Input: part model. Units: mm. Frame: model coordinates. A direction names the side the tool comes from. Coordinates: 2 decimals unless noted, no trailing zeros. Write each loop counter-clockwise with the first axis right and the second up, starting at its lowest first coordinate (ties: lowest second). Pieces come first, ordered by that corner, then holes. Notation, with made-up numbers: (-9.5, 11) -> (28.5, 11) arc R22 cw to (28.5, 34) -> close; hole circle Ø7 at (32.25, 29.5). An arc over 180 degrees is marked (long way). Use one line per item in the form item = value. Start each with the question number.
(1) Cut plane C-C on x = 5. Return the cut outline in (y, z) (3 decimals), plus the area to 3 significant figures.
(2) First-contact query: pin 1 (3 mm diameter, centred on x = 130, y = -77, fed in from +Z); pin 2 (9.5 mm diameter, centred on x = -242.5, z = 11, fed in from +Y); pin 3 (2 mm diameter, centred on x = 47.5, z = 30, fed in from -Y) (3 decimals); pin 4 (10 mm diameter, centred on x = 128, y = 30, fed in from -Z). Flat tips, straight axial feed; report the tip coordinate or a pass-through.
(3) Cut plane D-D on y = 0. Return the cut outline in (x, z).
(4) Cut plane B-B on x = 252. Return the cut outline in (y, z) (3 decimals), plus the area to 3 significant figures.
(5) Set-up query: faces 1 (the face through (-236, -92, 3.302)), 2 (the face through (-238.123, -85.516, 9.741)), 3 (the face through (177.8, 114, 28)). Return all of +Z, -Z, +X, -X, +Y, -Y with unobstructed straight access to the full face (end or side cutting, diameter ignored); none if empty.
(6) Ray query, line 1 along X through (y, z) = (92.5, 15.5); line 2 along Y through (x, z) = (-246, 2.5) (3 decimals); line 3 along X through (y, z) = (-50, 10.5). Return the intervals inside material, ascending.
(7) Pull-direction query (X, two-part tool) for faces 4 (the face through (166, 31.75, 21)), 5 (the face through (-4, 94, 0)); classes: released by +X, released by -X, zero draft, split by the parting line, or undercut.
(8) Cut plane A-A on x = 186.5. State how many separate pieces and enclosed holes the cut face has, plus the area to 3 significant figures.
```python
from build123d import *

# Parameters (mm, degrees)
F0_W         = 609.6
F0_H         = 241.3
F1_DEPTH     = 38.1
F3_DEPTH     = 38.101
F4_W         = 76.2
F4_H         = 50.8
F5_DEPTH     = 19.05
F6_R         = 12.7
F8_DEPTH     = 88.9
F10_DEPTH    = 88.9
F11_W        = 609.6
F11_H        = 66.675
F12_DEPTH    = 22.098
F13_W        = 609.6
F13_H        = 63.5
F14_DEPTH    = 11.049
F15_W        = 101.6
F15_H        = 191.5146559477
F16_DEPTH    = 19.05
F17_T1_DEPTH = 19.05
F17_T3_DEPTH = 16.002
F18_W        = 20.32
F18_H        = 3.302
F19_DEPTH    = 609.601


# Not quite as in the source:
# - a fillet or chamfer that OpenCascade refuses, or shapes differently, is made with other operations: its cross-section is extruded or revolved along the edge and cut away or added
# - a pattern or mirror of a feature is missing from the dataset's text; its kind, count and spacing are read off the source's solid


with BuildPart() as f1:
    # F0 (on Top) → F1 (new body)
    with BuildSketch(Plane.XY):
        Rectangle(F0_W, F0_H)
    extrude(amount=F1_DEPTH)

    # F2 (on face) → F3 (cut, through all)
    with BuildSketch(Plane.XY.offset(38.1)):
        with BuildLine():
            Line((-101.6, -76.2), (-228.6, -76.2))
            ThreePointArc((-228.6, -76.2), (-238.125, -85.725), (-228.6, -95.25))
            Line((-228.6, -95.25), (-101.6, -95.25))
            ThreePointArc((-101.6, -95.25), (-92.075, -85.725), (-101.6, -76.2))
        make_face()
        with BuildLine():
            Line((-228.6, -31.75), (-101.6, -31.75))
            ThreePointArc((-101.6, -31.75), (-92.075, -22.225), (-101.6, -12.7))
            Line((-101.6, -12.7), (-228.6, -12.7))
            ThreePointArc((-228.6, -12.7), (-238.125, -22.225), (-228.6, -31.75))
        make_face()
        with BuildLine():
            Line((-228.6, 31.75), (-101.6, 31.75))
            ThreePointArc((-101.6, 31.75), (-92.075, 41.275), (-101.6, 50.8))
            Line((-101.6, 50.8), (-228.6, 50.8))
            ThreePointArc((-228.6, 50.8), (-238.125, 41.275), (-228.6, 31.75))
        make_face()
    f3 = extrude(amount=-F3_DEPTH, mode=Mode.SUBTRACT)

    # F3_copies: F3 across plane
    add(f3.mirror(Plane(origin=(0, 0, 0), x_dir=(0, 0, 1), z_dir=(1, 0, 0))), mode=Mode.SUBTRACT)

    # F4 (on face) → F5 (cut)
    with BuildSketch(Plane(origin=(0, 0, 0), x_dir=(1, 0, 0), z_dir=(0, 0, -1))):
        with Locations((241.3, -95.25)):
            Rectangle(F4_W, F4_H)
    f5 = extrude(amount=-F5_DEPTH, mode=Mode.SUBTRACT)

    # F5_copies: F5 across plane
    add(f5.mirror(Plane(origin=(0, 0, 0), x_dir=(0, 0, -1), z_dir=(-1, 0, 0))), mode=Mode.SUBTRACT)

    # F6
    f6_edges = [f1.edges().sort_by_distance(p)[0] for p in [
        (279.4, 69.85, 9.525),
        (203.2, 69.85, 9.525),
    ]]
    fillet(f6_edges, radius=F6_R)

    # F7 (on Right) → F8 (cut, symmetric)
    with BuildSketch(Plane.YZ):
        Polygon((120.65, 38.1), (110.4411357684, 38.1), (120.65, 0), align=None)
    extrude(amount=F8_DEPTH, both=True, mode=Mode.SUBTRACT)

    # F9 (on face) → F10 (cut)
    with BuildSketch(Plane.YZ.offset(-88.9)):
        Polygon((98.6529547439, 38.1), (120.65, 0), (120.65, 38.1), align=None)
    f10 = extrude(amount=-F10_DEPTH, mode=Mode.SUBTRACT)

    # F10_copies: F10 across plane
    add(f10.mirror(Plane(origin=(0, 0, 0), x_dir=(0, 0, 1), z_dir=(1, 0, 0))), mode=Mode.SUBTRACT)

    # F11 (on face) → F12 (cut)
    with BuildSketch(Plane.XY.offset(38.1)):
        with Locations((0, -87.3125)):
            Rectangle(F11_W, F11_H)
    extrude(amount=-F12_DEPTH, mode=Mode.SUBTRACT)

    # F13 (on face) → F14 (cut)
    with BuildSketch(Plane.XY.offset(38.1)):
        with Locations((0, -22.225)):
            Rectangle(F13_W, F13_H)
    extrude(amount=-F14_DEPTH, mode=Mode.SUBTRACT)

    # F15 (on face) → F16 (cut)
    with BuildSketch(Plane(origin=(0, 0, 0), x_dir=(1, 0, 0), z_dir=(0, 0, -1))):
        with Locations((0, 6.5381005406)):
            Rectangle(F15_W, F15_H)
    extrude(amount=-F16_DEPTH, mode=Mode.SUBTRACT)

    # F17: fillet of radius 12.7 on 6 edges, made by hand

    # F17_s2 → F17_t1 (join)
    with BuildSketch(Plane.XY):
        with BuildLine():
            ThreePointArc((-50.8004, 76.5182617478), (-47.0802561211, 85.4994835543), (-38.0990343146, 89.2196274332))
            Line((-38.0990343146, 89.2196274332), (-38.0990343146, 90.4897640017))
            ThreePointArc((-38.0990343146, 90.4897640017), (-44.4495171573, 90.4893640017), (-50.8, 90.4893640017))
            Line((-50.8, 90.4893640017), (-52.0701365685, 89.2192274332))
            ThreePointArc((-52.0701365685, 89.2192274332), (-52.0701365685, 82.8687445905), (-52.0705365685, 76.5182617478))
            Line((-52.0705365685, 76.5182617478), (-50.8004, 76.5182617478))
        make_face()
        with BuildLine():
            ThreePointArc((50.8004, 76.5182617478), (47.0802561211, 85.4994835543), (38.0990343146, 89.2196274332))
            Line((38.0990343146, 89.2196274332), (38.0990343146, 90.4897640017))
            ThreePointArc((38.0990343146, 90.4897640017), (44.4495171573, 90.4893640017), (50.8, 90.4893640017))
            Line((50.8, 90.4893640017), (52.0701365685, 89.2192274332))
            ThreePointArc((52.0701365685, 89.2192274332), (52.0701365685, 82.8687445905), (52.0705365685, 76.5182617478))
            Line((52.0705365685, 76.5182617478), (50.8004, 76.5182617478))
        make_face()
        with BuildLine():
            ThreePointArc((-203.1996, 82.5509656854), (-206.9197438789, 73.5697438789), (-215.9009656854, 69.8496))
            Line((-215.9009656854, 69.8496), (-215.9009656854, 68.5794634315))
            ThreePointArc((-215.9009656854, 68.5794634315), (-209.5504828427, 68.5798634315), (-203.2, 68.5798634315))
            Line((-203.2, 68.5798634315), (-201.9298634315, 69.85))
            ThreePointArc((-201.9298634315, 69.85), (-201.9298634315, 76.2004828427), (-201.9294634315, 82.5509656854))
            Line((-201.9294634315, 82.5509656854), (-203.1996, 82.5509656854))
        make_face()
        with BuildLine():
            ThreePointArc((-266.6990343146, 69.8496), (-275.6802561211, 73.5697438789), (-279.4004, 82.5509656854))
            Line((-279.4004, 82.5509656854), (-280.6705365685, 82.5509656854))
            ThreePointArc((-280.6705365685, 82.5509656854), (-280.6701365685, 76.2004828427), (-280.6701365685, 69.85))
            Line((-280.6701365685, 69.85), (-279.4, 68.5798634315))
            ThreePointArc((-279.4, 68.5798634315), (-273.0495171573, 68.5798634315), (-266.6990343146, 68.5794634315))
            Line((-266.6990343146, 68.5794634315), (-266.6990343146, 69.8496))
        make_face()
    extrude(amount=F17_T1_DEPTH)

    # F17_s4 → F17_t3 (join)
    with BuildSketch(Plane.XY):
        with BuildLine():
            ThreePointArc((-50.8004, -89.5944628291), (-47.0802561211, -98.5756846355), (-38.0990343146, -102.2958285145))
            Line((-38.0990343146, -102.2958285145), (-38.0990343146, -103.565965083))
            ThreePointArc((-38.0990343146, -103.565965083), (-44.4495171573, -103.565565083), (-50.8, -103.565565083))
            Line((-50.8, -103.565565083), (-52.0701365685, -102.2954285145))
            ThreePointArc((-52.0701365685, -102.2954285145), (-52.0701365685, -95.9449456718), (-52.0705365685, -89.5944628291))
            Line((-52.0705365685, -89.5944628291), (-50.8004, -89.5944628291))
        make_face()
        with BuildLine():
            ThreePointArc((38.0990343146, -102.2958285145), (47.0802561211, -98.5756846355), (50.8004, -89.5944628291))
            Line((50.8004, -89.5944628291), (52.0705365685, -89.5944628291))
            ThreePointArc((52.0705365685, -89.5944628291), (52.0701365685, -95.9449456718), (52.0701365685, -102.2954285145))
            Line((52.0701365685, -102.2954285145), (50.8, -103.565565083))
            ThreePointArc((50.8, -103.565565083), (44.4495171573, -103.565565083), (38.0990343146, -103.565965083))
            Line((38.0990343146, -103.565965083), (38.0990343146, -102.2958285145))
        make_face()
    extrude(amount=F17_T3_DEPTH)

    # F18 (on face) → F19 (cut, through all)
    with BuildSketch(Plane(origin=(-304.8, 0, 0), x_dir=(0, -1, 0), z_dir=(-1, 0, 0))):
        with Locations((-41.275, 1.651)):
            Rectangle(F18_W, F18_H)
        with Locations((22.225, 1.651)):
            Rectangle(F18_W, F18_H)
        with Locations((85.725, 1.651)):
            Rectangle(F18_W, F18_H)
    extrude(amount=-F19_DEPTH, mode=Mode.SUBTRACT)


solid = f1.part
```
Values:
q1.outline = (-120.65, 0) -> (-102.295, 0) -> (-102.295, 16.002) -> (-120.65, 16.002) -> close; (-53.975, 19.05) -> (89.219, 19.05) -> (89.219, 0) -> (120.65, 0) -> (110.441, 38.1) -> (9.525, 38.1) -> (9.525, 27.051) -> (-53.975, 27.051) -> close
q1.area = 3,320 mm2
q2.pin_1 = 16
q2.pin_2 = 69.85
q2.pin_3 = 9.525
q2.pin_4 = 0
q3.outline = (-304.8, 0) -> (-50.8, 0) -> (-50.8, 19.05) -> (50.8, 19.05) -> (50.8, 0) -> (304.8, 0) -> (304.8, 27.05) -> (-304.8, 27.05) -> close
q4.outline = (-120.65, 0) -> (-95.885, 0) -> (-95.885, 3.302) -> (-75.565, 3.302) -> (-75.565, 0) -> (-32.385, 0) -> (-32.385, 3.302) -> (-12.065, 3.302) -> (-12.065, 0) -> (31.115, 0) -> (31.115, 3.302) -> (51.435, 3.302) -> (51.435, 0) -> (69.85, 0) -> (69.85, 19.05) -> (120.65, 19.05) -> (120.65, 38.1) -> (9.525, 38.1) -> (9.525, 27.051) -> (-53.975, 27.051) -> (-53.975, 16.002) -> (-120.65, 16.002) -> close
q4.area = 5,850 mm2
q5.face_1 = -Z, +X, -X
q5.face_2 = +Z, -Z
q5.face_3 = +Z, +Y
q6.line_1 = -304.8 to -279.4, -203.2 to 203.2, 279.4 to 304.8
q6.line_2 = -120.65 to -95.885, -75.565 to -32.385, -12.065 to 31.115, 51.435 to 69.85
q6.line_3 = -304.8 to -50.8, 50.8 to 304.8
q7.face_4 = undercut
q7.face_5 = zero draft
q8.separate_pieces = 4
q8.enclosed_holes = 0
q8.area = 5,460 mm2
